from build123d import *


with BuildPart() as f1:
    # F0 (on Front) → F1 (revolve)
    with BuildSketch(Plane.XZ):
        with BuildLine():
            Line((0, 44.45), (0, 0))
            Line((0, 0), (0, -2.54))
            Line((0, -2.54), (6.6654079201, -2.54))
            Line((6.6654079201, -2.54), (6.6654079201, 0))
            Line((6.6654079201, 0), (4.1254079201, 0))
            add(Edge.make_bspline(
                [(2.7243491478, 37.01434877), (2.9172660711, 35.6191618602), (2.8364055922, 32.1757037693), (1.0664201554, 27.9096087669), (4.4148443102, 16.489578027), (4.4669372205, 4.8023526907), (4.1254079201, 2.1266304433), (4.1254079201, 0)],
                knots=[0.0802289089, 0.0802289089, 0.0802289089, 0.0802289089, 0.1899326983, 0.3516504376, 0.5980111539, 0.8398924382, 1, 1, 1, 1], degree=3))
            add(Edge.make_bspline(
                [(1.9050000945, 40.0049999055), (2.3215219262, 39.0568329152), (2.5832645566, 38.0346811043), (2.7243491478, 37.01434877)],
                knots=[0, 0, 0, 0, 0.0802289089, 0.0802289089, 0.0802289089, 0.0802289089], degree=3))
            Line((1.9050000945, 40.0049999055), (0.3574084009, 41.9613287769))
            ThreePointArc((0.3574084009, 41.9613287769), (1.257102723, 43.360537675), (0, 44.45))
        make_face()
        with BuildLine():
            Line((3.8100001889, 38.0999998111), (1.9050000945, 40.0049999055))
            add(Edge.make_bspline(
                [(1.9050000945, 40.0049999055), (2.3215219262, 39.0568329152), (2.5832645566, 38.0346811043), (2.7243491478, 37.01434877)],
                knots=[0, 0, 0, 0, 0.0802289089, 0.0802289089, 0.0802289089, 0.0802289089], degree=3))
            Line((2.7243491478, 37.01434877), (3.8100001889, 38.0999998111))
        make_face()
    revolve(axis=Axis((0, 0, 22.225), (0, 0, 1)))


solid = f1.part
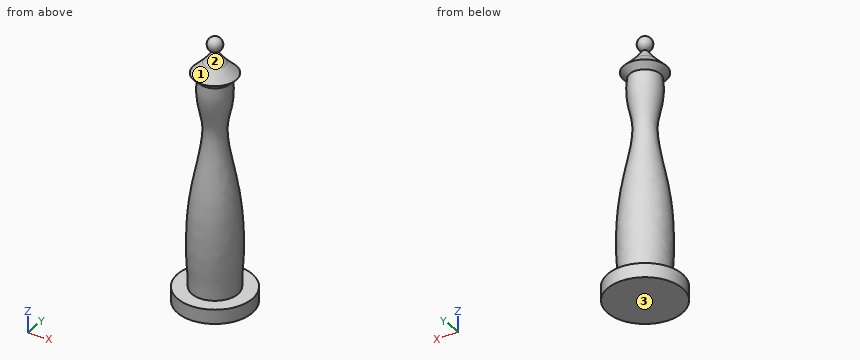
Read the model definition and answer for the solid it produces. Units are mm, in the model's axes. Face numbers are marked on the shaded views. Coordinates: 2 decimals unless noted, no trailing zeros. Order: outer loops, then holes, each group sorted by start corner. A loop starts at its lowest first (then second) coordinate and runs counter-clockwise, first axis right, second up. Notation, with made-up numbers: (83, -1) - (117, -1) arc R27 cw to (117, 29) - close; hole circle Ø4 at (2, 74.5). An arc over 180 degrees is marked (long way). Use one line per item in the form item = value.
(1) Section A-A, the plane x = 5.75 is taken. Give the vertices of the cut face in (y, z), then the cut area to 3 significant figures.
Computed values:
outline = (-3.37, -2.54) - (3.37, -2.54) - (3.37, 0) - (-3.37, 0) - close
area = 17.1 mm²
(2) Section B-B, the plane x = -6 is taken. Give the vertices of the cut face in (y, z), then the cut area to 3 significant figures.
Computed values:
outline = (-2.9, -2.54) - (2.9, -2.54) - (2.9, 0) - (-2.9, 0) - close
area = 14.7 mm²
(3) Given pin 1 Ø3 at (x, z) = (2.5, 4.5) entering from +Y; pin 2 Ø4 at (x, z) = (1.5, 9.5) entering from +Y; pin 3 Ø1 at (y, z) = (0.5, 19) entering from -X, each flat-ended and moving along its own axis, determine where each tip first touches the part or whether it passes through.
Computed values:
pin_1 = 4.21
pin_2 = 4.39
pin_3 = -3.43
(4) For a pull along Z with two mould halves and no side action, classify the marked faces 1, 2 and 3 as pulls with the +Z half, pulls with the -Z half, needs draft (parallel to the pull), parting line crosses it, or undercut.
Computed values:
face_1 = pulls with the +Z half
face_2 = undercut
face_3 = pulls with the -Z half
(5) Straight lines are drawn through the part: L1, parallel to Z at x = -3.5, y = -5.5; L2, parallel to Z at x = 1, y = 0; L3, parallel to Y at x = -1.5, z = 38. For each, find the intervals that lie inside material, in ascending order.
Computed values:
L1 = -2.54 to 0
L2 = -2.54 to 41.15, 42.4 to 43.96
L3 = -3.39 to 3.39
